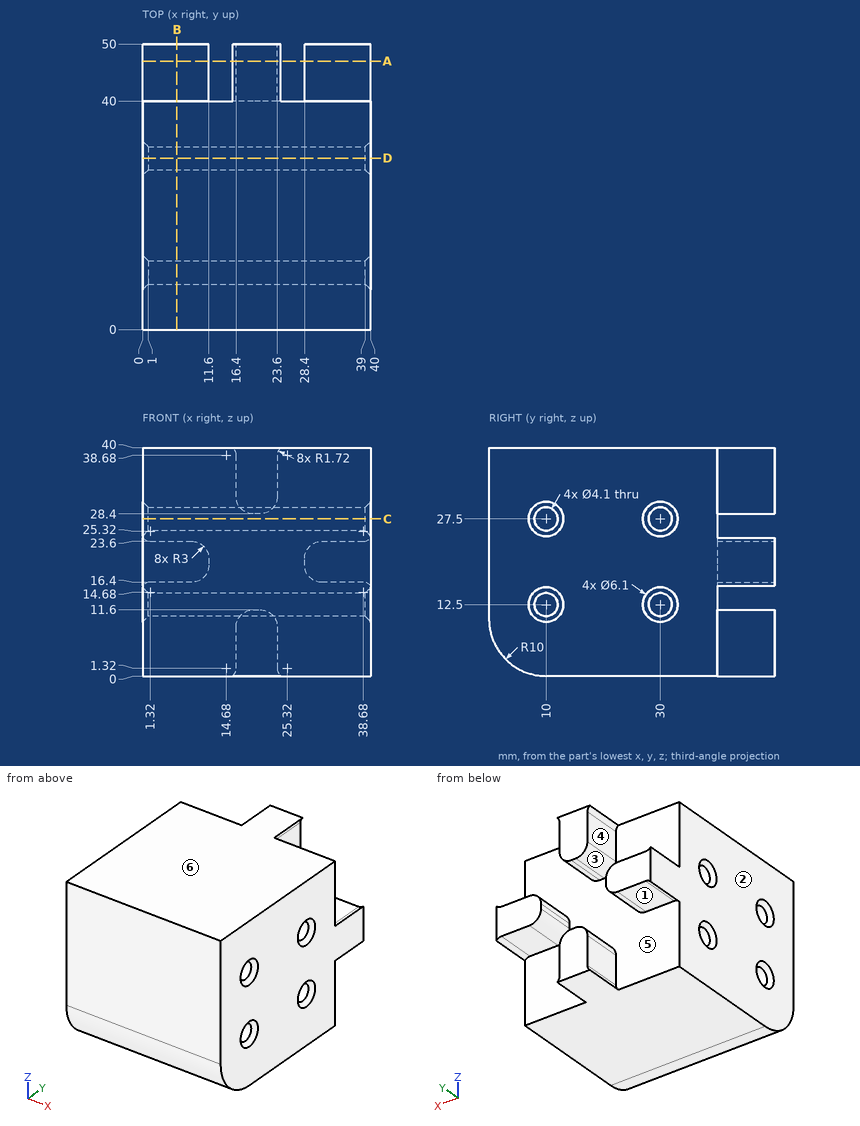
Verification items for this drawing (mm, ordinates from the low corner). A direction names the side the tool comes from. Round coordinates to 2 decimals unless told otherwise and drop trailing zeros. Loops run counter-clockwise (first coordinate to the right, second up) from the corner with the lowest first, then second, coordinate; pieces in that order, holes last. Notation, with made-up numbers: M 36,13.25 L 82,13.25 A33 ccw 82,41.25 Z; hole C 30,-21 d5. An arc over 180 degrees is marked long. Answer as a JSON object with one key per item and string values.
1. Access from +Z, -Z, +X, -X, +Y, -Y to the whole of each face (thin tool, end or side, straight path). Record for the marked faces 1, 2 and 3.
Reply:
{"face 1": "-Z, +Y", "face 2": "+Z, -Z, -X, +Y, -Y", "face 3": "-X, +Y"}
2. Section check A-A (y = 47). State how many separate pieces and enclosed holes the cut face has, plus the area to 3 significant figures.
Reply:
{"separate pieces": "4", "enclosed holes": "0", "area": "321 mm²"}
3. Scan lines: line 1 (Z direction, x = 10, y = 30); line 2 (Y direction, x = 20.5, z = 27.5); line 3 (Z direction, x = 21, y = 9). Record each from-to range of solid material in increasing order.
Reply:
{"line 1": "z = 0 to 10.45, 14.55 to 25.45, 29.55 to 40", "line 2": "y = 0 to 7.95, 12.05 to 27.95, 32.05 to 40", "line 3": "z = 0.05 to 10.71, 14.29 to 25.71, 29.29 to 40"}
4. Mould release check, pull along X, two halves, no side actions. Record for the marked faces 4, 5 and 6: pulls with the +X half, pulls with the -X half, needs draft (parallel to the pull), parting line crosses it, or undercut.
Reply:
{"face 4": "pulls with the -X half", "face 5": "undercut", "face 6": "needs draft"}
5. Section check C-C (z = 27.5). Record the boundary of the cut face in (x, y), plus the area to 3 significant figures.
Reply:
{"outline": "M 0,0 L 40,0 L 40,6.95 L 39,7.95 L 1,7.95 L 0,6.95 Z; M 0,13.05 L 1,12.05 L 39,12.05 L 40,13.05 L 40,26.95 L 39,27.95 L 1,27.95 L 0,26.95 Z; M 0,33.05 L 1,32.05 L 39,32.05 L 40,33.05 L 40,40 L 0,40 Z", "area": "1,270 mm²"}
6. Section check D-D (y = 30). Record the boundary of the cut face in (x, z).
Reply:
{"outline": "M 0,0 L 40,0 L 40,9.45 L 39,10.45 L 1,10.45 L 0,9.45 Z; M 0,15.55 L 1,14.55 L 39,14.55 L 40,15.55 L 40,24.45 L 39,25.45 L 1,25.45 L 0,24.45 Z; M 0,30.55 L 1,29.55 L 39,29.55 L 40,30.55 L 40,40 L 0,40 Z"}
7. Gauge pin test, flat ends, axial feed: P1, Ø5.5, axis at y = 30, z = 12.5, coming from the -X side; P2, Ø3.5, axis at y = 47, z = 5.5, coming from the -X side; P3, Ø6, axis at x = 35.5, y = 45, coming from the +Z side. Record the tip position at first contact, or that the pin passes through.
Reply:
{"P1": "stops at x = 0.3", "P2": "stops at x = 16.4", "P3": "stops at z = 23.6"}
8. Section check B-B (x = 6). Record the boundary of the cut face in (y, z), plus the area to 3 significant figures.
Reply:
{"outline": "M 0,10 A10 ccw 10,0 L 40,0 L 40,16.4 L 50,16.4 L 50,23.6 L 40,23.6 L 40,40 L 0,40 Z; hole C 10,12.5 d4.1; hole C 10,27.5 d4.1; hole C 30,12.5 d4.1; hole C 30,27.5 d4.1", "area": "1,600 mm²"}
